Here's how the part is built. I have some questions about the finished solid (model axes, mm). Face numbers are marked on the shaded views. A direction names the side the tool comes from. Give positions to 0.01 mm unless a question says otherwise; leave off trailing zeros. Write each loop counter-clockwise with the first axis right and the second up, starting at its lowest first coordinate (ties: lowest second). Pieces come first, ordered by that corner, then holes. Notation, with made-up numbers: (41.25, -10.5) - (60.25, -10.5) arc R22 ccw to (60.25, 15.5) - close; hole circle Ø3 at (17, 69). An arc over 180 degrees is marked (long way). Write each question's results on one line, items separated by ' | '. Start each with the question number.
Item 1: We'd pull the mould along X, two halves only. Please class the marked faces 1 and 2: +X half, -X half, draft (parallel to the pull), parting line (faces both ways), or undercut.
Item 2: Suppose I cut it at B-B on z = -3. List the corners of the cut face in (x, y) for me.
Item 3: Suppose I cut it at A-A on y = 2.5. Count the separate pieces of the cut face and the enclosed holes in it, then the cut area to 3 significant figures.
Item 4: Please list where these lines run through material, in increasing order: line 1 along X through (y, z) = (-2.7, 0); line 2 along X through (y, z) = (5, -33); line 3 along Y through (x, z) = (13, -19).
Item 5: Suppose I cut it at D-D on x = -11. List the corners of the cut face in (y, z) for me, then the cut area to 3 significant figures.
Item 6: Will these pins go through, and if not, where does the flat tip stop? P1, Ø2, axis at x = 20, y = 5, coming from the +Z side; P2, Ø8, axis at x = 8, z = 8.5, coming from the +Y side; P3, Ø4, axis at x = 27, z = 30, coming from the -Y side; P4, Ø4, axis at y = 1, z = -19.5, coming from the +X side.
Item 7: Which directions (+Z, -Z, +X, -X, +Y, -Y) give clear straight access to the entire face, cutting with the end or side of a thin tool? Please do the marked faces 3, 4 and 5.
Item 8: Suppose I cut it at C-C on z = 24.5. List the corners of the cut face in (x, y) for me (3 decimals).
```python
from build123d import *

# Parameters (mm, degrees)
SKETCH1_R              = 5
BOSS_EXTRUDE1_DEPTH    = 10
BOSS_EXTRUDE1_2_DEPTH  = 10
BOSS_EXTRUDE1_3_DEPTH  = 10
BOSS_EXTRUDE1_4_DEPTH  = 10
BOSS_EXTRUDE1_5_DEPTH  = 10
BOSS_EXTRUDE1_6_DEPTH  = 10
BOSS_EXTRUDE1_7_DEPTH  = 10
BOSS_EXTRUDE1_8_DEPTH  = 10
BOSS_EXTRUDE1_9_DEPTH  = 10
BOSS_EXTRUDE1_10_DEPTH = 10
BOSS_EXTRUDE1_11_DEPTH = 10
SKETCH2_R              = 35
SKETCH2_R_2            = 4
BOSS_EXTRUDE2_DEPTH    = 5
SKETCH3_W              = 0.25
SKETCH3_H              = 1.939339828
CUT_EXTRUDE1_DEPTH     = 0.1


with BuildPart() as part:
    # Sketch1 → Boss-Extrude1 (new body)
    with BuildSketch(Plane(origin=(0, 0, 0), x_dir=(1, 0, 0), z_dir=(0, 1, 0))):
        with Locations(Location((0, 35, 0), (0, 0, 270))):
            Circle(SKETCH1_R)
    extrude(amount=BOSS_EXTRUDE1_DEPTH)



with BuildPart() as body_2:
    # Sketch1 → Boss-Extrude1 2 (new body)
    with BuildSketch(Plane(origin=(0, 0, 0), x_dir=(1, 0, 0), z_dir=(0, 1, 0))):
        with Locations(Location((18.922428611, 29.443873649, 0), (0, 0, 270))):
            Circle(SKETCH1_R)
    extrude(amount=BOSS_EXTRUDE1_2_DEPTH)


with BuildPart() as body_3:
    # Sketch1 → Boss-Extrude1 3 (new body)
    with BuildSketch(Plane(origin=(0, 0, 0), x_dir=(1, 0, 0), z_dir=(0, 1, 0))):
        with Locations(Location((31.837119837, 14.539525455, 0), (0, 0, 270))):
            Circle(SKETCH1_R)
    extrude(amount=BOSS_EXTRUDE1_3_DEPTH)


with BuildPart() as body_4:
    # Sketch1 → Boss-Extrude1 4 (new body)
    with BuildSketch(Plane(origin=(0, 0, 0), x_dir=(1, 0, 0), z_dir=(0, 1, 0))):
        with Locations(Location((34.643750466, -4.98101934, 0), (0, 0, 270))):
            Circle(SKETCH1_R)
    extrude(amount=BOSS_EXTRUDE1_4_DEPTH)


with BuildPart() as body_5:
    # Sketch1 → Boss-Extrude1 5 (new body)
    with BuildSketch(Plane(origin=(0, 0, 0), x_dir=(1, 0, 0), z_dir=(0, 1, 0))):
        with Locations(Location((26.451235102, -22.920125688, 0), (0, 0, 270))):
            Circle(SKETCH1_R)
    extrude(amount=BOSS_EXTRUDE1_5_DEPTH)


with BuildPart() as body_6:
    # Sketch1 → Boss-Extrude1 6 (new body)
    with BuildSketch(Plane(origin=(0, 0, 0), x_dir=(1, 0, 0), z_dir=(0, 1, 0))):
        with Locations(Location((9.860639489, -33.582254077, 0), (0, 0, 270))):
            Circle(SKETCH1_R)
    extrude(amount=BOSS_EXTRUDE1_6_DEPTH)


with BuildPart() as body_7:
    # Sketch1 → Boss-Extrude1 7 (new body)
    with BuildSketch(Plane(origin=(0, 0, 0), x_dir=(1, 0, 0), z_dir=(0, 1, 0))):
        with Locations(Location((-9.860639489, -33.582254077, 0), (0, 0, 270))):
            Circle(SKETCH1_R)
    extrude(amount=BOSS_EXTRUDE1_7_DEPTH)


with BuildPart() as body_8:
    # Sketch1 → Boss-Extrude1 8 (new body)
    with BuildSketch(Plane(origin=(0, 0, 0), x_dir=(1, 0, 0), z_dir=(0, 1, 0))):
        with Locations(Location((-26.451235102, -22.920125688, 0), (0, 0, 270))):
            Circle(SKETCH1_R)
    extrude(amount=BOSS_EXTRUDE1_8_DEPTH)


with BuildPart() as body_9:
    # Sketch1 → Boss-Extrude1 9 (new body)
    with BuildSketch(Plane(origin=(0, 0, 0), x_dir=(1, 0, 0), z_dir=(0, 1, 0))):
        with Locations(Location((-34.643750466, -4.98101934, 0), (0, 0, 270))):
            Circle(SKETCH1_R)
    extrude(amount=BOSS_EXTRUDE1_9_DEPTH)


with BuildPart() as body_10:
    # Sketch1 → Boss-Extrude1 10 (new body)
    with BuildSketch(Plane(origin=(0, 0, 0), x_dir=(1, 0, 0), z_dir=(0, 1, 0))):
        with Locations(Location((-31.837119837, 14.539525455, 0), (0, 0, 270))):
            Circle(SKETCH1_R)
    extrude(amount=BOSS_EXTRUDE1_10_DEPTH)


with BuildPart() as body_11:
    # Sketch1 → Boss-Extrude1 11 (new body)
    with BuildSketch(Plane(origin=(0, 0, 0), x_dir=(1, 0, 0), z_dir=(0, 1, 0))):
        with Locations(Location((-18.922428611, 29.443873649, 0), (0, 0, 270))):
            Circle(SKETCH1_R)
    extrude(amount=BOSS_EXTRUDE1_11_DEPTH)


with BuildPart() as part_1:
    add(part.part)

    add(body_2.part)  # Boss-Extrude2 merges body 2

    add(body_3.part)  # Boss-Extrude2 merges body 3

    add(body_4.part)  # Boss-Extrude2 merges body 4

    add(body_5.part)  # Boss-Extrude2 merges body 5

    add(body_6.part)  # Boss-Extrude2 merges body 6

    add(body_7.part)  # Boss-Extrude2 merges body 7

    add(body_8.part)  # Boss-Extrude2 merges body 8

    add(body_9.part)  # Boss-Extrude2 merges body 9

    add(body_10.part)  # Boss-Extrude2 merges body 10

    add(body_11.part)  # Boss-Extrude2 merges body 11
    # Sketch2 → Boss-Extrude2 (add)
    with BuildSketch(Plane(origin=(0, 0, 0), x_dir=(1, 0, 0), z_dir=(0, 1, 0))):
        with Locations(Location((0, 0, 0), (0, 0, 270))):
            Circle(SKETCH2_R)
        with Locations(Location((0, 0, 0), (0, 0, 270))):
            Circle(SKETCH2_R_2, mode=Mode.SUBTRACT)
    extrude(amount=-BOSS_EXTRUDE2_DEPTH)

    # Sketch3 → Cut-Extrude1 (cut)
    with BuildSketch(Plane(origin=(0, 10, 0), x_dir=(1, 0, 0), z_dir=(0, 1, 0))):
        Polygon((-1.060660172, 36.939339828), (-0.25, 36.939339828), (-0.25, 37.75), align=None)
        Polygon((-0.25, 36.939339828), (0, 36.939339828), (0, 38), (-0.25, 37.75), align=None)
        Polygon((0, 38), (0, 36.939339828), (0.25, 36.939339828), (0.25, 37.75), align=None)
        Polygon((0.25, 37.75), (0.25, 36.939339828), (1.060660172, 36.939339828), align=None)
        with Locations((0.125, 35.969669914)):
            Rectangle(SKETCH3_W, SKETCH3_H)
        with Locations((-0.125, 35.969669914)):
            Rectangle(SKETCH3_W, SKETCH3_H)
    extrude(amount=-CUT_EXTRUDE1_DEPTH, mode=Mode.SUBTRACT)


solid = part_1.part
```
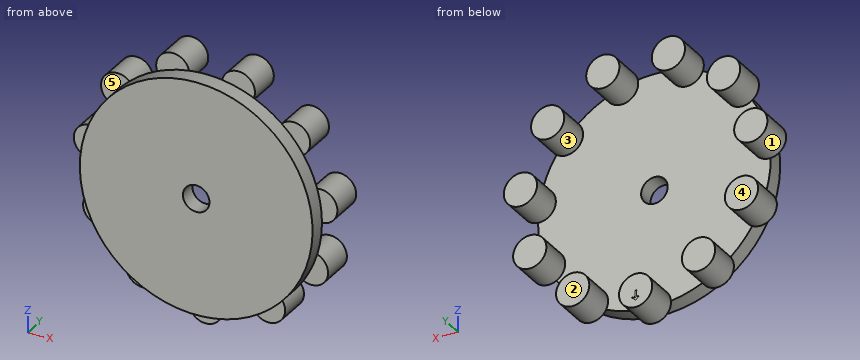
Checked values:
1) face 1: undercut | face 2: draft
2) outline: (-34.87, -5) - (-2.65, -5) - (-2.65, 0) - (-34.87, 0) - close; (2.65, -5) - (34.87, -5) - (34.87, 0) - (2.65, 0) - close
3) separate pieces: 11 | enclosed holes: 0 | area: 864 mm^2
4) line 1: x = -35 to -4, 4 to 35 | line 2: x = -22.44 to -15.41, -4.58 to 4.58, 15.41 to 22.44 | line 3: y = -5 to 0
5) outline: (-5, -33.23) - (0, -33.23) - (0, 28.71) - (10, 28.71) - (10, 38.45) - (0, 38.45) - (0, 33.23) - (-5, 33.23) - close | area: 430 mm^2
6) P1: stops at z = -24.44 | P2: stops at y = 0 | P3: passes through | P4: stops at x = 35.87
7) face 3: +Y | face 4: +Z, -Z, +X, -X, +Y | face 5: +Z, -X, -Y
8) outline: (-31.195, 0) - (-24.995, 0) - (-24.995, -5) - (24.995, -5) - (24.995, 0) - (31.195, 0) - (31.195, 10) - (21.707, 10) - (21.707, 0) - (-21.707, 0) - (-21.707, 10) - (-31.195, 10) - close
